Work out the finished part from the listing and answer in its coordinate system (mm). A direction names the side the tool comes from. Round coordinates to 2 decimals unless told otherwise and drop trailing zeros. Order: outer loops, then holes, each group sorted by start corner. A loop starts at its lowest first (then second) coordinate and runs counter-clockwise, first axis right, second up. Notation, with made-up numbers: (1.5, 85) - (18.5, 85) arc R13 ccw to (18.5, 107) - close; hole circle Ø6 at (-12, 85.25). An arc over 180 degrees is marked (long way). Use CSV: the item, a comma, the result in double quotes.
from build123d import *

# Parameters (mm, degrees)
SKETCH_1_R          = 12.2
EXTRUDE_1_DEPTH     = 43.8
SKETCH_3_R          = 1.5
CUT_EXTRUDE_1_DEPTH = 4
CHAMFER_1_SIZE      = 0.85
CHAMFER_1_SIZE2     = 2.3
SKETCH_4_R          = 6.4
EXTRUDE_2_DEPTH     = 1.5
SKETCH_5_R          = 6
EXTRUDE_3_DEPTH     = 0.4
SKETCH_6_R          = 5
EXTRUDE_4_DEPTH     = 0.7
SKETCH_7_R          = 3
EXTRUDE_5_DEPTH     = 14.4
SKETCH_8_R          = 1.5
CUT_EXTRUDE_2_DEPTH = 5.5
CUT_EXTRUDE_3_DEPTH = 11.5
SKETCH_10_R         = 1.5
CUT_EXTRUDE_4_DEPTH = 15.7
CUT_EXTRUDE_START   = -13
SKETCH_11_R         = 12.2
SKETCH_11_R_2       = 7
CUT_EXTRUDE_5_DEPTH = 0.6
EXTRUDE_6_REACH     = 32.9
SKETCH_12_W         = 8
SKETCH_12_H         = 1.5
SKETCH_13_R         = 1
CUT_EXTRUDE_6_DEPTH = 3
SKETCH_14_R         = 3
EXTRUDE_7_DEPTH     = 4
CHAMFER_2_SIZE      = 0.2
CHAMFER_2_SIZE2     = 0.1


with BuildPart() as part:
    # 草图1 → 凸台-拉伸1 (new body)
    with BuildSketch(Plane(origin=(0, 0, 0), x_dir=(1, 0, 0), z_dir=(0, 1, 0))):
        Circle(SKETCH_1_R)
    extrude(amount=EXTRUDE_1_DEPTH)

    # 草图3 → 切除-拉伸1 (cut)
    with BuildSketch(Plane(origin=(0, 43.8, 0), x_dir=(1, 0, 0), z_dir=(0, 1, 0))):
        with Locations((0, 9.5)):
            Circle(SKETCH_3_R)
        with Locations((-8.227241336, -4.75)):
            Circle(SKETCH_3_R)
        with Locations((8.227241336, -4.75)):
            Circle(SKETCH_3_R)
    extrude(amount=-CUT_EXTRUDE_1_DEPTH, mode=Mode.SUBTRACT)

    # 倒角1
    chamfer_1_edges = [part.edges().sort_by_distance(p)[0] for p in [
        (-12.2, 0, 0),
    ]]
    chamfer_1_side = [part.faces().sort_by_distance(p)[0] for p in [
        (0, 0, 0),
    ]]
    chamfer(chamfer_1_edges, length=CHAMFER_1_SIZE, length2=CHAMFER_1_SIZE2, reference=chamfer_1_side[0])

    # 草图4 → 凸台-拉伸2 (add)
    with BuildSketch(Plane(origin=(0, 43.8, 0), x_dir=(1, 0, 0), z_dir=(0, 1, 0))):
        Circle(SKETCH_4_R)
    extrude(amount=EXTRUDE_2_DEPTH)

    # 草图5 → 凸台-拉伸3 (add)
    with BuildSketch(Plane(origin=(0, 45.3, 0), x_dir=(1, 0, 0), z_dir=(0, 1, 0))):
        Circle(SKETCH_5_R)
    extrude(amount=EXTRUDE_3_DEPTH)

    # 草图6 → 凸台-拉伸4 (add)
    with BuildSketch(Plane(origin=(0, 45.7, 0), x_dir=(1, 0, 0), z_dir=(0, 1, 0))):
        Circle(SKETCH_6_R)
    extrude(amount=EXTRUDE_4_DEPTH)

    # 草图7 → 凸台-拉伸5 (add)
    with BuildSketch(Plane(origin=(0, 46.4, 0), x_dir=(1, 0, 0), z_dir=(0, 1, 0))):
        Circle(SKETCH_7_R)
    extrude(amount=EXTRUDE_5_DEPTH)

    # 草图8 → 切除-拉伸2 (cut)
    with BuildSketch(Plane(origin=(0, 60.8, 0), x_dir=(1, 0, 0), z_dir=(0, 1, 0))):
        Circle(SKETCH_8_R)
    extrude(amount=-CUT_EXTRUDE_2_DEPTH, mode=Mode.SUBTRACT)

    # 草图9 → 切除-拉伸3 (cut)
    with BuildSketch(Plane(origin=(0, 60.8, 0), x_dir=(1, 0, 0), z_dir=(0, 1, 0))):
        with BuildLine():
            Line((-1.658312395, -2.5), (1.658312395, -2.5))
            ThreePointArc((1.658312395, -2.5), (0, -3), (-1.658312395, -2.5))
        make_face()
    extrude(amount=-CUT_EXTRUDE_3_DEPTH, mode=Mode.SUBTRACT)

    # 草图10 → 切除-拉伸4 (cut, through all)
    with BuildSketch(Plane.XY.offset(2.5)):
        with Locations((0, 51.8)):
            Circle(SKETCH_10_R)
    extrude(amount=-CUT_EXTRUDE_4_DEPTH, mode=Mode.SUBTRACT)

    # 草图11 → 切除-拉伸5 (cut)
    with BuildSketch(Plane.XZ.offset(CUT_EXTRUDE_START)):
        Circle(SKETCH_11_R)
        Circle(SKETCH_11_R_2, mode=Mode.SUBTRACT)
    extrude(amount=-CUT_EXTRUDE_5_DEPTH, mode=Mode.SUBTRACT)

    # 草图12 → 凸台-拉伸6 (add, up to next)
    with BuildSketch(Plane(origin=(18.7, 0, 0), x_dir=(0, 0, -1), z_dir=(1, 0, 0)), mode=Mode.PRIVATE) as extrude_6_sk1:
        with Locations((0, 14.35)):
            Rectangle(SKETCH_12_W, SKETCH_12_H)
    extrude_6_tool1 = extrude(extrude_6_sk1.sketch, amount=-EXTRUDE_6_REACH, mode=Mode.PRIVATE) - part.part
    add(extrude_6_tool1.solids().sort_by_distance((18.7, 14.35, 0))[0])

    # 草图13 → 切除-拉伸6 (cut)
    with BuildSketch(Plane.XZ):
        with Locations((0, 5.5)):
            Circle(SKETCH_13_R)
        with Locations((-4.763139721, -2.75)):
            Circle(SKETCH_13_R)
        with Locations((4.763139721, -2.75)):
            Circle(SKETCH_13_R)
    extrude(amount=-CUT_EXTRUDE_6_DEPTH, mode=Mode.SUBTRACT)

    # 草图14 → 凸台-拉伸7 (add)
    with BuildSketch(Plane.XZ):
        Circle(SKETCH_14_R)
    extrude(amount=EXTRUDE_7_DEPTH)

    # 倒角2
    chamfer_2_edges = [part.edges().sort_by_distance(p)[0] for p in [
        (-3, -4, 0),
    ]]
    chamfer_2_side = [part.faces().sort_by_distance(p)[0] for p in [
        (-3, -2, 0),
    ]]
    chamfer(chamfer_2_edges, length=CHAMFER_2_SIZE, length2=CHAMFER_2_SIZE2, reference=chamfer_2_side[0])


solid = part.part
(1) For faces 4 (the cylindrical face through (-0.13, 1.48, 6.49)), 5 (the cylindrical face through (0, 42, -8)), 6 (the flat face through (15, 14, -4)), determine the directions among +Z, -Z, +X, -X, +Y, -Y from which every point of the face is accessible in a straight line to the end or side of a thin tool.
Findings below:
face 4,"-Y"
face 5,"+Y"
face 6,"-Z, +X, +Y, -Y"
(2) Find the intervals of material crossed by L1, parallel to Z at x = 0, y = 56.65; L2, parallel to Y at x = 7.5, z = -1.5; L3, parallel to Y at x = 9, z = 6, in increasing order. Write a range as from..to.
Findings below:
L1,"z = -3..-1.5, 1.5..2.5"
L2,"y = 0..13, 13.6..43.8"
L3,"y = 0..13, 13.6..39.8"
(3) Each of these flat-tipped pins is pushed along its axis until it touches: pin 1 (5.5 mm diameter, centred on x = 15, z = 1, fed in from +Y); pin 2 (7.5 mm diameter, centred on x = 5, z = 5.5, fed in from -Y); pin 3 (4 mm diameter, centred on y = 28.5, z = -7.5, fed in from -X). Where does it stop, or does it pass through?
Findings below:
pin 1,"stops at y = 15.1"
pin 2,"stops at y = 0"
pin 3,"stops at x = -10.89"
(4) The mould has two halves that part along X. Classify faces 1 (the cylindrical face through (-1.08, 46.05, 4.88)), 2 (the flat face through (0, -4, 0)), 3 (the flat face through (-8, 39.8, 5)): released by +X, released by -X, zero draft, split by the parting line, or undercut.
Findings below:
face 1,"split by the parting line"
face 2,"zero draft"
face 3,"undercut"
(5) Find section B-B (y = 24). Determine the outline of the cut face in (x, z).
Findings below:
outline,"circle Ø24.4 at (0, 0)"
(6) Find section A-A (y = 51.8). Determine the outline of the cut face in (x, z), and give its area (3 significant figures).
Findings below:
outline,"(-1.66, 2.5) arc R3 ccw to (-1.5, -2.6) - (-1.5, 2.5) - close; (1.5, -2.6) arc R3 ccw to (1.66, 2.5) - (1.5, 2.5) - close"
area,"11.0 mm²"
